Here's the drawing with two shaded views (mm, measured from the low corner). I have some questions. A direction names the side the tool comes from. Coordinates: 2 decimals unless noted, no trailing zeros. Order: outer loops, then holes, each group sorted by start corner. A loop starts at its lowest first (then second) coordinate and runs counter-clockwise, first axis right, second up. Notation, with made-up numbers: (-33.5, 4) -> (5.5, 4) arc R28 ccw to (5.5, 38) -> close; hole circle Ø2 at (39, 20). An arc over 180 degrees is marked (long way). Answer as a JSON object with one key per item and string values. Group by question number.
(1) I want a section at C-C, the plane y = 30. List the corners of the cut face in (x, z) for me (1 decimal).
(2) I need wall thicknesses on line 1 (Y direction, x = 63, z = 26) (1 decimal); line 2 (X direction, y = 46.5, z = 41) (1 decimal); line 3 (Z direction, x = 39.5, y = 33). Which ranges of each line are inside material? Lowest first, please.
(3) For pin 1 (10 mm diameter, centred on y = 30.5, z = 36.5, fed in from +X) (1 decimal); pin 2 (4 mm diameter, centred on x = 65, y = 28, fed in from +Z); pin 3 (3 mm diameter, centred on x = 30.5, y = 43, fed in from +Z), each with a flat end and sliding along its axis, tell me the tip position at first contact or that it passes through.
(4) I want a section at B-B, the plane x = 56. List the corners of the cut face in (y, z) for me (1 decimal).
(5) Which directions (+Z, -Z, +X, -X, +Y, -Y) give clear straight access to the entire face, cutting with the end or side of a thin tool? Please do the marked faces 4, 5 and 6.
(6) I want a section at A-A, the plane z = 44. List the corners of the cut face in (x, y) for me (1 decimal).
(7) If we mould it in two halves opening along Y, with no side actions, what happens to the marked faces 1, 2 and 3? For each: pulls with the +Y half, pulls with the -Y half, needs draft (parallel to the pull), parting line crosses it, or undercut.
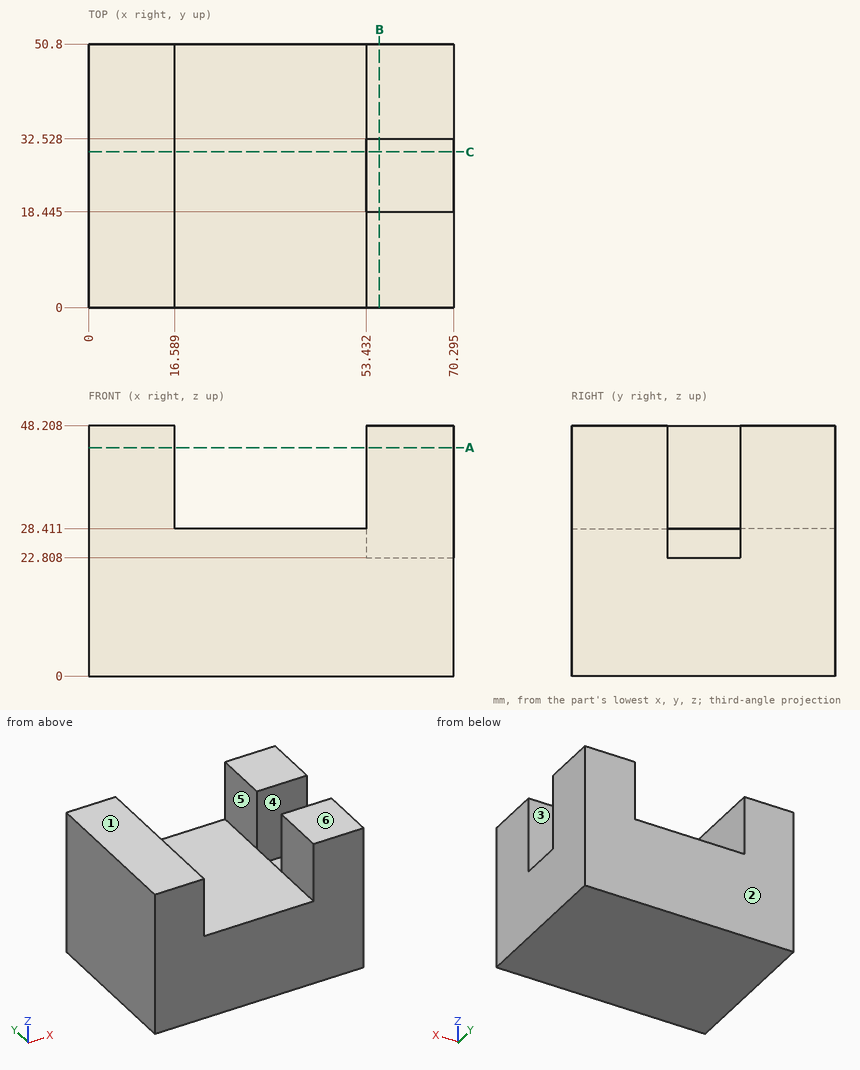
Computed values:
{
 "1": {"outline": "(0, 0) -> (70.3, 0) -> (70.3, 22.8) -> (53.4, 22.8) -> (53.4, 28.4) -> (16.6, 28.4) -> (16.6, 48.2) -> (0, 48.2) -> close"},
 "2": {"line 1": "y = 0 to 18.4, 32.5 to 50.8", "line 2": "x = 0 to 16.6, 53.4 to 70.3", "line 3": "z = 0 to 28.41"},
 "3": {"pin 1": "stops at x = 70.3", "pin 2": "stops at z = 22.81", "pin 3": "stops at z = 28.41"},
 "4": {"outline": "(0, 0) -> (50.8, 0) -> (50.8, 48.2) -> (32.5, 48.2) -> (32.5, 22.8) -> (18.4, 22.8) -> (18.4, 48.2) -> (0, 48.2) -> close"},
 "5": {"face 4": "+Z, +X", "face 5": "+Z, +Y, -Y", "face 6": "+Z, +X, -X, +Y, -Y"},
 "6": {"outline": "(0, 0) -> (16.6, 0) -> (16.6, 50.8) -> (0, 50.8) -> close; (53.4, 0) -> (70.3, 0) -> (70.3, 18.4) -> (53.4, 18.4) -> close; (53.4, 32.5) -> (70.3, 32.5) -> (70.3, 50.8) -> (53.4, 50.8) -> close"},
 "7": {"face 1": "needs draft", "face 2": "pulls with the +Y half", "face 3": "undercut"}
}
